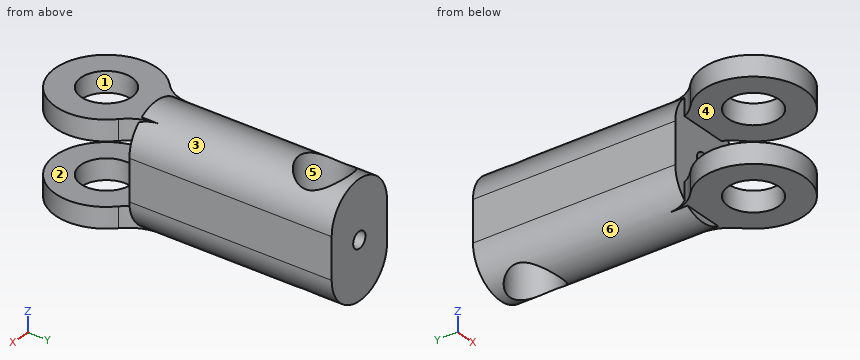
from build123d import *

# Parameters (mm, degrees)
BOSS_EXTRUDE1_START     = 7.5
SKETCH1_R               = 6.25
BOSS_EXTRUDE1_DEPTH     = 5
BOSS_EXTRUDE2_START     = -7.5
SKETCH1_2_R             = 6.25
BOSS_EXTRUDE2_DEPTH     = 5
BOSS_EXTRUDE3_START     = 12.5
BOSS_EXTRUDE3_DEPTH     = 50
SKETCH3_R               = 2
CUT_EXTRUDE1_DEPTH      = 56
CUT_EXTRUDE2_DEPTH      = 47
CUT_EXTRUDE2_DEPTH_BACK = 29
SKETCH4_R               = 6.25


with BuildPart() as part:
    # Sketch1 → Boss-Extrude1 (new body)
    with BuildSketch(Plane.XY.offset(BOSS_EXTRUDE1_START)):
        with BuildLine():
            Line((5, 18.456439237), (-5, 18.456439237))
            Line((-5, 18.456439237), (-5, 16.770509831))
            ThreePointArc((-5, 16.770509831), (-5.871290708, 12.688026927), (-8.333333333, 9.316949906))
            ThreePointArc((-8.333333333, 9.316949906), (0, -12.5), (8.333333333, 9.316949906))
            ThreePointArc((8.333333333, 9.316949906), (5.871290708, 12.688026927), (5, 16.770509831))
            Line((5, 16.770509831), (5, 18.456439237))
        make_face()
        Circle(SKETCH1_R, mode=Mode.SUBTRACT)
    extrude(amount=BOSS_EXTRUDE1_DEPTH)



with BuildPart() as body_2:
    # Sketch1_2 → Boss-Extrude2 (new body)
    with BuildSketch(Plane.XY.offset(BOSS_EXTRUDE2_START)):
        with BuildLine():
            Line((5, 18.456439237), (-5, 18.456439237))
            Line((-5, 18.456439237), (-5, 16.770509831))
            ThreePointArc((-5, 16.770509831), (-5.871290708, 12.688026927), (-8.333333333, 9.316949906))
            ThreePointArc((-8.333333333, 9.316949906), (0, -12.5), (8.333333333, 9.316949906))
            ThreePointArc((8.333333333, 9.316949906), (5.871290708, 12.688026927), (5, 16.770509831))
            Line((5, 16.770509831), (5, 18.456439237))
        make_face()
        Circle(SKETCH1_2_R, mode=Mode.SUBTRACT)
    extrude(amount=-BOSS_EXTRUDE2_DEPTH)


with BuildPart() as part_1:
    add(part.part)

    add(body_2.part)  # Boss-Extrude3 merges body 2
    # Sketch2 → Boss-Extrude3 (add)
    with BuildSketch(Plane(origin=(0, 0, 0), x_dir=(1, 0, 0), z_dir=(0, 1, 0)).offset(BOSS_EXTRUDE3_START)):
        with BuildLine():
            Line((9.013878189, 5), (9.013878189, -5))
            ThreePointArc((9.013878189, -5), (0, -14.013878189), (-9.013878189, -5))
            Line((-9.013878189, -5), (-9.013878189, 5))
            ThreePointArc((-9.013878189, 5), (0, 14.013878189), (9.013878189, 5))
        make_face()
    extrude(amount=BOSS_EXTRUDE3_DEPTH)

    # Sketch3 → Cut-Extrude1 (cut)
    with BuildSketch(Plane.XZ.offset(-12.5)):
        with Locations(Location((0, 0, 0), (0, 0, 270))):
            Circle(SKETCH3_R)
    extrude(amount=-CUT_EXTRUDE1_DEPTH, mode=Mode.SUBTRACT)

    # Sketch4 → Cut-Extrude2 (cut, two sides: drawn at the far end of the back side and taken through both)
    with BuildSketch(Plane.XY.offset(-CUT_EXTRUDE2_DEPTH_BACK)):
        with Locations(Location((0, 53.915919761, 0), (0, 0, 180))):
            Circle(SKETCH4_R)
    extrude(amount=CUT_EXTRUDE2_DEPTH + CUT_EXTRUDE2_DEPTH_BACK, mode=Mode.SUBTRACT)


solid = part_1.part
Build history of the part. All positions in model axes, mm. Face numbers are marked on the shaded views. A direction names the side the tool comes from. Give positions to 0.01 mm unless a question says otherwise; leave off trailing zeros. Loops run counter-clockwise (first coordinate to the right, second up) from the corner with the lowest first, then second, coordinate; pieces in that order, holes last. Notation, with made-up numbers: (-21.5, 22) -> (3.5, 22) arc R11 ccw to (3.5, 39) -> close; hole circle Ø7 at (-13.5, 6). An arc over 180 degrees is marked (long way). Answer in a Markdown table with one row per item.
Item 1: Slice it at B-B on x = 0. Give the number of separate pieces and of enclosed holes in the cut face, plus the area to 3 significant figures.
Findings below:
| item | result |
|---|---|
| separate pieces | 6 |
| enclosed holes | 0 |
| area | 1,030 mm² |
Item 2: Probe line 1 along Y through (x, z) = (0, 9.2); line 2 along Z through (x, y) = (-6, 3); line 3 along Y through (x, z) = (-1.5, 9.25). List the from-to ranges inside material, lowest first. Write a range as [from, to].
Findings below:
| item | result |
|---|---|
| line 1 | y = [-12.5, -6.25], [6.25, 47.67], [60.17, 62.5] |
| line 2 | z = [-12.5, -7.5], [7.5, 12.5] |
| line 3 | y = [-12.41, -6.07], [6.07, 47.85], [59.98, 62.5] |
Item 3: Slice it at C-C on z = 0.75. Write the cut outline in (x, y), plus the area to 3 significant figures.
Findings below:
| item | result |
|---|---|
| outline | (-9.01, 12.5) -> (-1.85, 12.5) -> (-1.85, 47.95) arc R6.25 cw to (-1.85, 59.88) -> (-1.85, 62.5) -> (-9.01, 62.5) -> close; (1.85, 12.5) -> (9.01, 12.5) -> (9.01, 62.5) -> (1.85, 62.5) -> (1.85, 59.88) arc R6.25 cw to (1.85, 47.95) -> close |
| area | 639 mm² |
Item 4: Mould opens along X. For the marked faces 1, 2 and 3 say: pulls with the +X half, pulls with the -X half, needs draft (parallel to the pull), parting line crosses it, or undercut.
Findings below:
| item | result |
|---|---|
| face 1 | undercut |
| face 2 | needs draft |
| face 3 | parting line crosses it |
Item 5: Slice it at D-D on z = -10.5. Write the cut outline in (x, y), plus the area to 3 significant figures.
Findings below:
| item | result |
|---|---|
| outline | (-8.33, 9.32) arc R12.5 ccw (long way) to (8.33, 9.32) arc R10 cw to (5.96, 12.5) -> (7.14, 12.5) -> (7.14, 62.5) -> (-7.14, 62.5) -> (-7.14, 12.5) -> (-5.96, 12.5) arc R10 cw to start; hole circle Ø12.5 at (0, 0); hole circle Ø12.5 at (0, 53.92) |
| area | 968 mm² |
Item 6: Tool access for the marked faces 4, 5 and 6: list every direction of +Z, -Z, +X, -X, +Y, -Y with a clear straight run to the whole face (end or side of a thin tool).
Findings below:
| item | result |
|---|---|
| face 4 | +X, -X, -Y |
| face 5 | +Z, -Z |
| face 6 | -Z, +Y |
Item 7: Slice it at A-A on y = -7.5. Write the cut outline in (x, z).
Findings below:
| item | result |
|---|---|
| outline | (-10, -12.5) -> (10, -12.5) -> (10, -7.5) -> (-10, -7.5) -> close; (-10, 7.5) -> (10, 7.5) -> (10, 12.5) -> (-10, 12.5) -> close |
Item 8: Flat gauge pins, fed straight in: P1, Ø12, axis at x = -4, y = 2, coming from the -Z side; P2, Ø2.5, axis at x = 0, z = 0, coming from the -Y side; P3, Ø5, axis at y = 33.5, z = 2, coming from the -X side; P4, Ø10, axis at y = 18, z = 11, coming from the +X side. Where does each tip first touch, or does it go through?
Findings below:
| item | result |
|---|---|
| P1 | stops at z = -12.5 |
| P2 | passes through |
| P3 | stops at x = -9.01 |
| P4 | stops at x = 8.96 |
